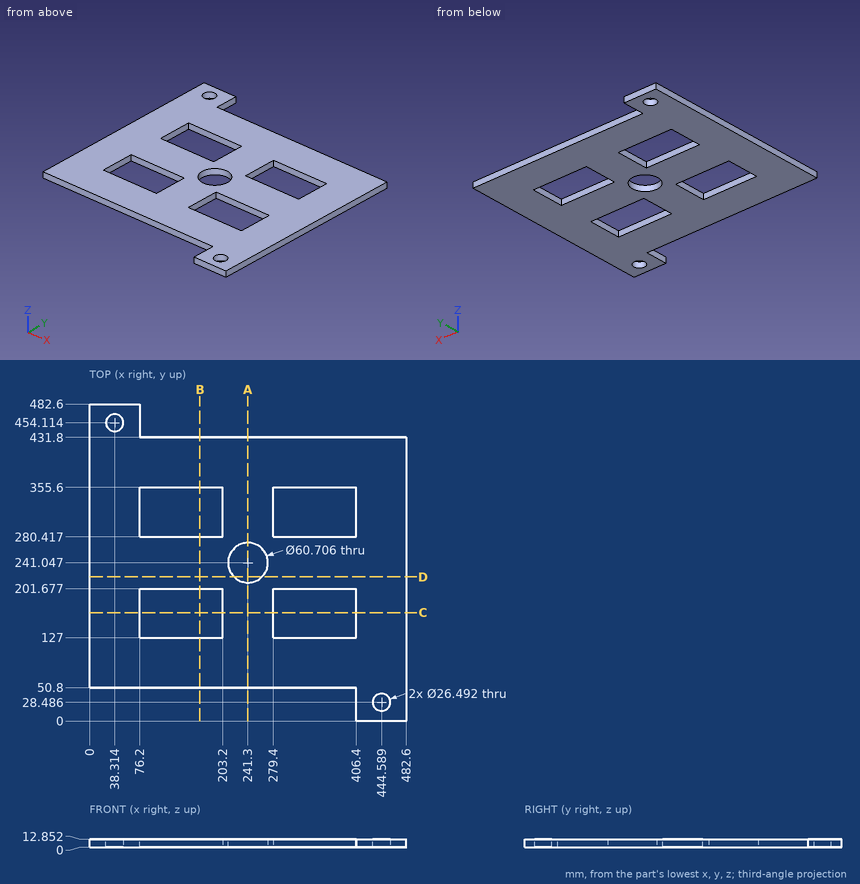
Print and shaded views of the part. All mm, measured from the part's lowest x, y and z. Round coordinates to 2 decimals unless told otherwise and drop trailing zeros. Write each loop counter-clockwise with the first axis right and the second up, starting at its lowest first coordinate (ties: lowest second). Pieces come first, ordered by that corner, then holes. Notation, with made-up numbers: (-36, 9) -> (-1, 9) arc R12 cw to (-1, 15) -> close; hole circle Ø7 at (-6, -5). An arc over 180 degrees is marked (long way). Return JSON: item names as keys, results as strings. Group by question number.
Q1. Saw through at B-B on x = 168. Write the cut outline in (y, z), plus the area to 3 significant figures.
Q2. Saw through at A-A on x = 241.3. Write the cut outline in (y, z).
Q3. Saw through at C-C on y = 165. Write the cut outline in (x, z), plus the area to 3 significant figures.
Q4. Probe L1, parallel to Y at x = 382, z = 7.5; L2, parallel to X at y = 150, z = 2.75; L3, parallel to Y at x = 241.3, z = 5.5. List the from-to ranges inside material, lowest first. Write a range as [from, to].
Q5. Pin check, flat tips, straight feed: pin 1 (4 mm diameter, centred on x = 246.5, z = 4.5, fed in from -Y); pin 2 (2 mm diameter, centred on x = 201.5, z = 2, fed in from +Y); pin 3 (4 mm diameter, centred on y = 14, z = 5, fed in from -X). Stop position of each tip, or through.
Q6. Saw through at D-D on y = 219.5. Write the cut outline in (x, z).
Answer:
{
 "1": {"outline": "(50.8, 0) -> (127, 0) -> (127, 12.85) -> (50.8, 12.85) -> close; (201.68, 0) -> (280.42, 0) -> (280.42, 12.85) -> (201.68, 12.85) -> close; (355.6, 0) -> (431.8, 0) -> (431.8, 12.85) -> (355.6, 12.85) -> close", "area": "2,970 mm2"},
 "2": {"outline": "(50.8, 0) -> (210.69, 0) -> (210.69, 12.85) -> (50.8, 12.85) -> close; (271.4, 0) -> (431.8, 0) -> (431.8, 12.85) -> (271.4, 12.85) -> close"},
 "3": {"outline": "(0, 0) -> (76.2, 0) -> (76.2, 12.85) -> (0, 12.85) -> close; (203.2, 0) -> (279.4, 0) -> (279.4, 12.85) -> (203.2, 12.85) -> close; (406.4, 0) -> (482.6, 0) -> (482.6, 12.85) -> (406.4, 12.85) -> close", "area": "2,940 mm2"},
 "4": {"L1": "[50.8, 127], [201.68, 280.42], [355.6, 431.8]", "L2": "[0, 76.2], [203.2, 279.4], [406.4, 482.6]", "L3": "[50.8, 210.69], [271.4, 431.8]"},
 "5": {"pin 1": "y = 50.8", "pin 2": "y = 431.8", "pin 3": "x = 406.4"},
 "6": {"outline": "(0, 0) -> (219.92, 0) -> (219.92, 12.85) -> (0, 12.85) -> close; (262.68, 0) -> (482.6, 0) -> (482.6, 12.85) -> (262.68, 12.85) -> close"}
}
